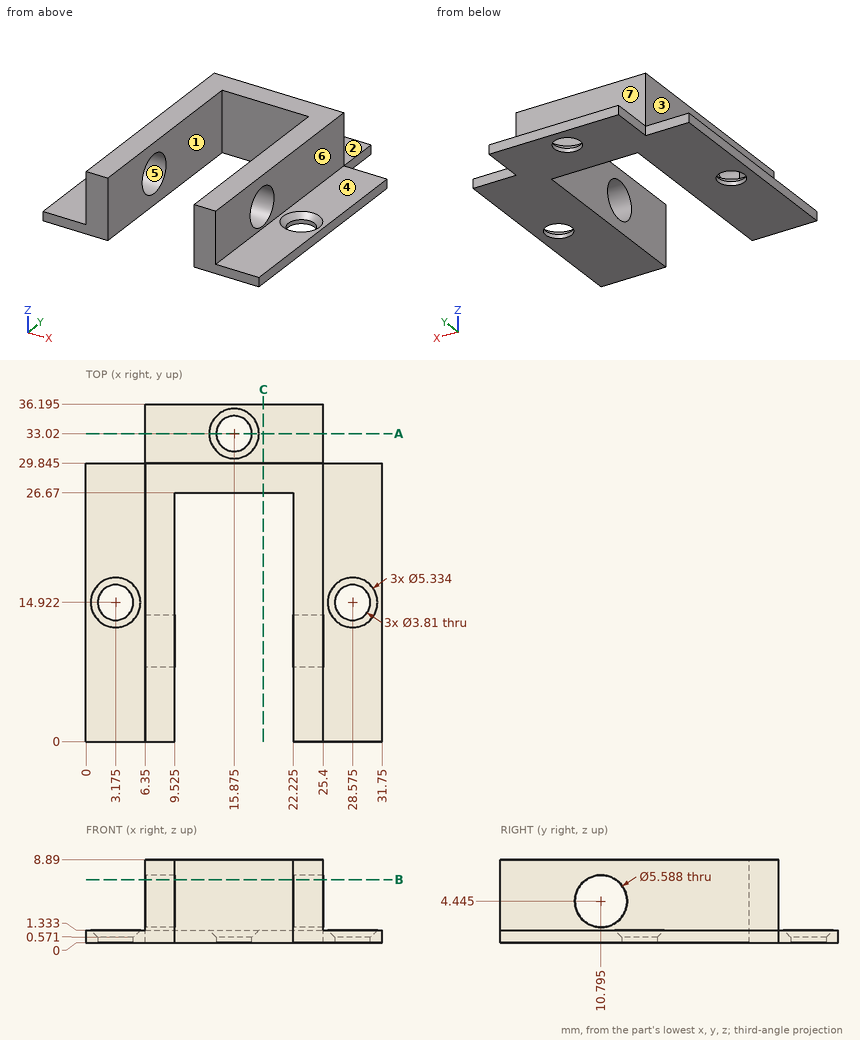
Check sheet for the drawn part. Datum: minimum x, y, z corner. Units: mm. A direction names the side the tool comes from. Coordinates: 2 decimals unless noted, no trailing zeros. Order: outer loops, then holes, each group sorted by start corner. A loop starts at its lowest first (then second) coordinate and runs counter-clockwise, first axis right, second up. Notation, with made-up numbers: M 56.25,-18 L 71.25,-18 A19 ccw 71.25,9 Z; hole C 55,67.5 d4. An arc over 180 degrees is marked long. One line per question, with ' | ' between items. Start each with the question number.
Item 1: Material ranges on L1, parallel to Z at x = 26, y = 26; L2, parallel to Y at x = 18, z = 6.5 (1 decimal); L3, parallel to Y at x = 26, z = 1 (1 decimal), recorded low to high. Write a range as [from, to].
Item 2: Cross-section at A-A on y = 33.02. Enter the section's corners in (x, z).
Item 3: Gauge pin test, flat ends, axial feed: pin 1 (1.9 mm diameter, centred on x = 30, y = 14.5, fed in from +Z); pin 2 (0.7 mm diameter, centred on x = 28, z = 0.5, fed in from +Y) (1 decimal); pin 3 (4.5 mm diameter, centred on x = 17.5, z = 4, fed in from -Y). Record the tip position at first contact, or that the pin passes through.
Item 4: Cross-section at B-B on z = 6.75. State how many separate pieces and enclosed holes the cut face has, then the cut area to 3 significant figures.
Item 5: Draft check along Y on the marked faces 5, 6 and 7. Enter one of: pulls with the +Y half, pulls with the -Y half, needs draft (parallel to the pull), parting line crosses it, or undercut.
Item 6: Set-up check for the marked faces 1, 2, 3 and 4: record each of +Z, -Z, +X, -X, +Y, -Y from which the full face is reachable in a straight line by a thin tool's end or side.
Item 7: Cross-section at C-C on x = 19. Enter the section's corners in (y, z) (1 decimal).
Findings:
1) L1: z = [0, 1.33] | L2: y = [26.7, 29.8] | L3: y = [0, 29.8]
2) outline: M 6.35,0 L 13.97,0 L 13.97,0.57 L 13.21,1.33 L 6.35,1.33 Z; M 17.78,0 L 25.4,0 L 25.4,1.33 L 18.54,1.33 L 17.78,0.57 Z
3) pin 1: stops at z = 1.1 | pin 2: stops at y = 29.8 | pin 3: stops at y = 26.67
4) separate pieces: 3 | enclosed holes: 0 | area: 210 mm²
5) face 5: undercut | face 6: needs draft | face 7: pulls with the +Y half
6) face 1: +Z, -Z, -Y | face 2: +Z, +X, -X, +Y | face 3: +Z, -X, +Y, -Y | face 4: +Z, +X, +Y, -Y
7) outline: M 26.7,0 L 36.2,0 L 36.2,1.3 L 29.8,1.3 L 29.8,8.9 L 26.7,8.9 Z
